The model under review builds one solid part; all positions refer to its coordinate system, in mm. A direction names the side the tool comes from. Round coordinates to 2 decimals unless told otherwise and drop trailing zeros. Write each loop counter-clockwise with the first axis right and the second up, starting at its lowest first coordinate (ties: lowest second). Pieces come first, ordered by that corner, then holes. Notation, with made-up numbers: (64, -4) - (119, -4) arc R35 cw to (119, 31) - close; hole circle Ø8 at (46, -12.75). An arc over 180 degrees is marked (long way). Return JSON: item names as keys, results as strings.
from build123d import *

# Parameters (mm, degrees)
SKETCH1_W           = 100
SKETCH1_H           = 69.85
BOSS_EXTRUDE1_DEPTH = 7
SKETCH2_R           = 1.25
CUT_EXTRUDE1_DEPTH  = 4
SKETCH3_W           = 25
SKETCH3_H           = 61.85
SKETCH3_W_2         = 29.1
SKETCH3_W_3         = 6.5
CUT_EXTRUDE2_DEPTH  = 8
SKETCH4_W           = 61.85
SKETCH4_H           = 5
CUT_EXTRUDE3_DEPTH  = 94.5


with BuildPart() as part:
    # Sketch1 → Boss-Extrude1 (new body)
    with BuildSketch(Plane(origin=(0, 0, 0), x_dir=(1, 0, 0), z_dir=(0, 1, 0))):
        with Locations((50, 34.925)):
            Rectangle(SKETCH1_W, SKETCH1_H)
    extrude(amount=BOSS_EXTRUDE1_DEPTH)

    # Sketch2 → Cut-Extrude1 (cut)
    with BuildSketch(Plane.XY):
        with Locations((86, 3)):
            Circle(SKETCH2_R)
        with Locations((9.4, 3)):
            Circle(SKETCH2_R)
    cut_extrude1 = extrude(amount=-CUT_EXTRUDE1_DEPTH, mode=Mode.SUBTRACT)

    # Sketch3 → Cut-Extrude2 (cut, through all)
    with BuildSketch(Plane(origin=(0, 7, 0), x_dir=(1, 0, 0), z_dir=(0, 1, 0))):
        with Locations((29.4, 34.925)):
            Rectangle(SKETCH3_W, SKETCH3_H)
        with Locations((63.95, 34.925)):
            Rectangle(SKETCH3_W_2, SKETCH3_H)
        with Locations((96.75, 34.925)):
            Rectangle(SKETCH3_W_3, SKETCH3_H)
    extrude(amount=-CUT_EXTRUDE2_DEPTH, mode=Mode.SUBTRACT)

    # Sketch4 → Cut-Extrude3 (cut, through all)
    with BuildSketch(Plane(origin=(93.5, 0, 0), x_dir=(0, 0, -1), z_dir=(1, 0, 0))):
        with Locations((34.925, 4.5)):
            Rectangle(SKETCH4_W, SKETCH4_H)
    extrude(amount=-CUT_EXTRUDE3_DEPTH, mode=Mode.SUBTRACT)

    # Mirror1: Cut-Extrude1 across plane
    add(cut_extrude1.mirror(Plane.XY.offset(-34.925)), mode=Mode.SUBTRACT)


solid = part.part
(1) Add section A-A (z = -21). Write out the cut boundary in (x, y).
Filled in:
{"outline": "(0, 0) - (16.9, 0) - (16.9, 2) - (0, 2) - close; (41.9, 0) - (49.4, 0) - (49.4, 2) - (41.9, 2) - close; (78.5, 0) - (93.5, 0) - (93.5, 2) - (78.5, 2) - close"}
(2) Clearance check with flat-ended pins moving along their axes: pin 1 Ø1 at (y, z) = (1.5, -42.5) entering from +X; pin 2 Ø8.5 at (x, z) = (7.5, -22) entering from +Y; pin 3 Ø1.5 at (y, z) = (3, -40.5) entering from -X. State where each tip first meets the part, or that it passes through.
Filled in:
{"pin 1": "stops at x = 93.5", "pin 2": "stops at y = 2", "pin 3": "passes through"}
(3) Add section B-B (y = 3). Write out the cut boundary in (x, z).
Filled in:
{"outline": "(0, -69.85) - (8.15, -69.85) - (8.15, -65.85) - (0, -65.85) - close; (0, -4) - (8.15, -4) - (8.15, 0) - (0, 0) - close; (10.65, -69.85) - (84.75, -69.85) - (84.75, -65.85) - (10.65, -65.85) - close; (10.65, -4) - (84.75, -4) - (84.75, 0) - (10.65, 0) - close; (87.25, -69.85) - (100, -69.85) - (100, -65.85) - (87.25, -65.85) - close; (87.25, -4) - (100, -4) - (100, 0) - (87.25, 0) - close"}
(4) Add section D-D (x = 15). Write out the cut boundary in (y, z).
Filled in:
{"outline": "(0, -69.85) - (7, -69.85) - (7, -65.85) - (2, -65.85) - (2, -4) - (7, -4) - (7, 0) - (0, 0) - close"}
(5) Add section C-C (x = 59.5). Write out the cut boundary in (y, z).
Filled in:
{"outline": "(0, -69.85) - (7, -69.85) - (7, -65.85) - (0, -65.85) - close; (0, -4) - (7, -4) - (7, 0) - (0, 0) - close"}
(6) Wall thickness on line 1 (X direction, y = 3, z = -67.2); line 2 (X direction, y = 1.5, z = -40.5); line 3 (Y direction, x = 86, z = -68): over which ranges is each line inside the solid? List them lowest first.
Filled in:
{"line 1": "x = 0 to 8.15, 10.65 to 84.75, 87.25 to 100", "line 2": "x = 0 to 16.9, 41.9 to 49.4, 78.5 to 93.5", "line 3": "y = 0 to 1.75, 4.25 to 7"}
(7) For faces 1 (the flat face through (78.5, 1, -34)), 2 (the flat face through (51, 3, -4)), 3 (the cylindrical face through (10.072, 4.054, -1.972)), list the 3-axis set-ups (+Z, -Z, +X, -X, +Y, -Y) from which the entire face can be reached by the end or side of a thin tool; tool diameter is ignored.
Filled in:
{"face 1": "+Y, -Y", "face 2": "+Y", "face 3": "+Z"}
(8) Mouldability with a two-part tool opening along X and no side actions: class faces 4 (the flat face through (9, 2, -34)), 5 (the flat face through (0, 1, -27)), 6 (the cylindrical face through (10.072, 4.054, -67.878)) as released by +X, released by -X, zero draft, split by the parting line, or undercut.
Filled in:
{"face 4": "zero draft", "face 5": "released by -X", "face 6": "undercut"}
